The figure shows three views and two pictorial views of one solid part (mm, origin at its lowest corner). Answer the questions. A direction names the side the tool comes from. Give positions to 0.01 mm unless a question says otherwise; leave off trailing zeros. Write each loop counter-clockwise with the first axis right and the second up, starting at its lowest first coordinate (ties: lowest second). Pieces come first, ordered by that corner, then holes. Notation, with made-up numbers: M -27.75,6.5 L 15.25,6.5 A16 cw 15.25,32.5 Z; hole C 13.5,25 d9. An arc over 180 degrees is marked long. Return JSON: item names as keys, results as strings.
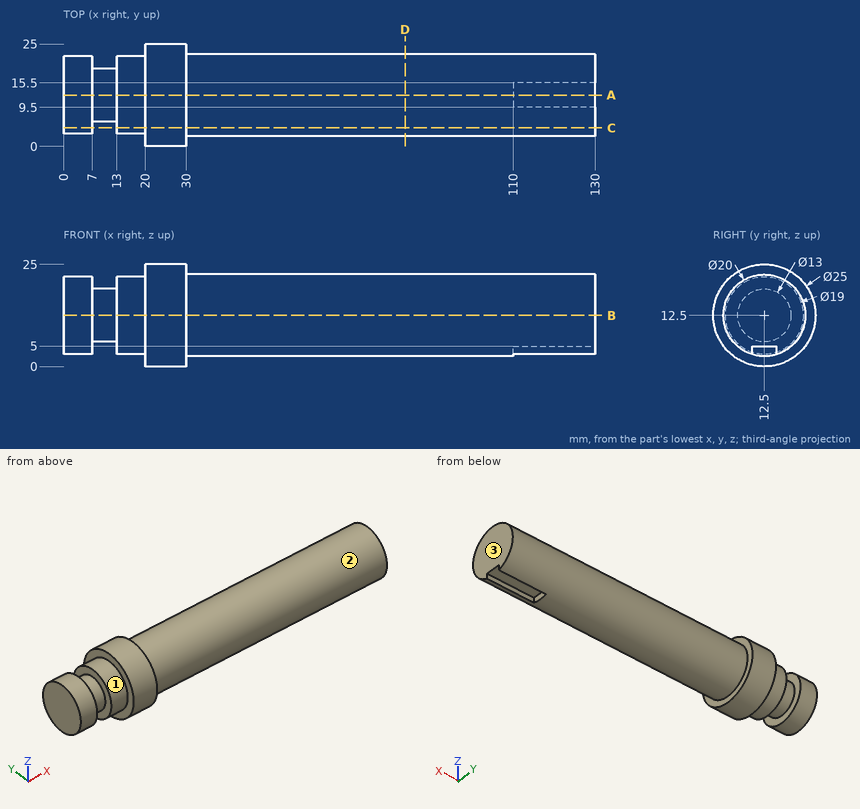
Item 1: A cutting plane is placed at A-A, the plane y = 12.5. Write down the section's boundary in (x, z), plus the area to 3 significant figures.
Geometry results:
{"outline": "M 0,3 L 7,3 L 7,6 L 13,6 L 13,3 L 20,3 L 20,0 L 30,0 L 30,2.5 L 110,2.5 L 110,5 L 130,5 L 130,22.5 L 30,22.5 L 30,25 L 20,25 L 20,22 L 13,22 L 13,19 L 7,19 L 7,22 L 0,22 Z", "area": "2,540 mm2"}
Item 2: A cutting plane is placed at C-C, the plane y = 4.5. Write down the section's boundary in (x, z), plus the area to 3 significant figures.
Geometry results:
{"outline": "M 0,7.38 L 7,7.38 L 7,17.62 L 0,17.62 Z; M 13,7.38 L 20,7.38 L 20,2.9 L 30,2.9 L 30,6.5 L 130,6.5 L 130,18.5 L 30,18.5 L 30,22.1 L 20,22.1 L 20,17.62 L 13,17.62 Z", "area": "1,540 mm2"}
Item 3: A cutting plane is placed at D-D, the plane x = 83.5. Write down the section's boundary in (y, z), plus the area to 3 significant figures.
Geometry results:
{"outline": "C 12.5,12.5 d20", "area": "314 mm2"}
Item 4: A cutting plane is placed at B-B, the plane z = 12.5. Write down the section's boundary in (x, y).
Geometry results:
{"outline": "M 0,3 L 7,3 L 7,6 L 13,6 L 13,3 L 20,3 L 20,0 L 30,0 L 30,2.5 L 130,2.5 L 130,22.5 L 30,22.5 L 30,25 L 20,25 L 20,22 L 13,22 L 13,19 L 7,19 L 7,22 L 0,22 Z"}
Item 5: Given pin 1 Ø8 at (x, y) = (65, 17.5) entering from +Z; pin 2 Ø8 at (x, y) = (95.5, 2.5) entering from +Z; pin 3 Ø12 at (y, z) = (21, 8) entering from -X; pin 4 Ø0.6 at (x, z) = (117, 4) entering from -Y, each flat-ended and moving along its own axis, determine where each tip first touches the part or whether it passes through.
Geometry results:
{"pin 1": "stops at z = 22.45", "pin 2": "stops at z = 20.5", "pin 3": "stops at x = 0", "pin 4": "stops at y = 6.78"}
Item 6: Find the intervals of material crossed by line 1 (X direction, y = 6.25, z = 6.75); line 2 (X direction, y = 10.5, z = 3.75); line 3 (Z direction, x = 18.5, y = 13), in increasing order.
Geometry results:
{"line 1": "x = 0 to 7, 13 to 130", "line 2": "x = 0 to 7, 13 to 110", "line 3": "z = 3.01 to 21.99"}
Item 7: Which of the six approach directions +Z, -Z, +X, -X, +Y, -Y give full straight-line access (tool end or side, diameter ignored) to the marked faces 1, 2 and 3?
Geometry results:
{"face 1": "-X", "face 2": "+X", "face 3": "+Z, -Z, +X, +Y, -Y"}
